Input: part model. Units: mm. Frame: model coordinates. A direction names the side the tool comes from. Coordinates: 2 decimals unless noted, no trailing zeros. Order: outer loops, then holes, each group sorted by start corner. A loop starts at its lowest first (then second) coordinate and runs counter-clockwise, first axis right, second up. Notation, with made-up numbers: M 19,-38 L 42,-38 A36 ccw 42,-2 Z; hole C -17.5,-22 d10. An arc over 180 degrees is marked long. One line per item, written item: value.
```python
from build123d import *

# Parameters (mm, degrees)
F0_W      = 55
F0_H      = 53.7
F0_R      = 2
F1_DEPTH  = 2
F2_DEPTH  = 4
F3_W      = 55
F3_H      = 27.5
F3_W_2    = 3.7
F3_H_2    = 2
F4_DEPTH  = 2
F5_START  = 1
F3_H_3    = 1.5
F5_DEPTH  = 1
F6_W      = 53.7
F6_H      = 27.5
F7_DEPTH  = 2
F8_START  = 1
F8_DEPTH  = 1
F10_DEPTH = 1.5
F11_W     = 55
F11_H     = 27.5
F11_W_2   = 3.7
F11_H_2   = 2
F12_DEPTH = 2
F13_START = 1
F13_DEPTH = 1
F15_DEPTH = 1.5
F16_W     = 1
F16_H     = 1.5
F16_W_2   = 53.7
F16_H_2   = 27.5
F17_DEPTH = 2
F18_START = 1
F18_DEPTH = 1
F20_DEPTH = 1.5
F21_W     = 1
F21_H     = 1
F22_DEPTH = 1.5
F23_R     = 0.3
F24_R     = 2
F25_R     = 0.5


with BuildPart() as f1:
    # F0 (on Top) → F1 (new body)
    with BuildSketch(Plane.XY):
        with Locations((27.5, 26.85)):
            Rectangle(F0_W, F0_H)
        with Locations((12, 11)):
            Circle(F0_R, mode=Mode.SUBTRACT)
        with Locations((43, 11)):
            Circle(F0_R, mode=Mode.SUBTRACT)
        with Locations((27.5, 46.7)):
            Circle(F0_R, mode=Mode.SUBTRACT)
    extrude(amount=F1_DEPTH)

    # F0 (on Top) → F2 (join)
    with BuildSketch(Plane.XY):
        with Locations((12, 11)):
            Circle(F0_R)
        with Locations((27.5, 46.7)):
            Circle(F0_R)
        with Locations((43, 11)):
            Circle(F0_R)
    extrude(amount=F2_DEPTH)

    # F3 (on face) → F4 (join)
    with BuildSketch(Plane.XZ):
        with Locations((27.5, 15.75)):
            Rectangle(F3_W, F3_H)
        with Locations((9.85, 26)):
            Rectangle(F3_W_2, F3_H_2, mode=Mode.SUBTRACT)
        with Locations((45.15, 26)):
            Rectangle(F3_W_2, F3_H_2, mode=Mode.SUBTRACT)
        with Locations((27.5, 1)):
            Rectangle(F3_W, F3_H_2)
    extrude(amount=F4_DEPTH)

    # F3 (on face) → F5 (join)
    with BuildSketch(Plane.XZ.offset(F5_START)):
        with Locations((27.5, 30.25)):
            Rectangle(F3_W, F3_H_3)
    extrude(amount=F5_DEPTH)

    # F6 (on face) → F7 (join)
    with BuildSketch(Plane.YZ.offset(55)):
        Polygon((-2, 29.5), (-2, 0), (53.7, 0), (53.7, 2), (0, 2), (0, 29.5), (-1, 29.5), align=None)
        with Locations((26.85, 15.75)):
            Rectangle(F6_W, F6_H)
        with BuildLine():
            ThreePointArc((23.7071067812, 9.7928932188), (22.2928932188, 9.7928932188), (22.2928932188, 11.2071067812))
            Line((22.2928932188, 11.2071067812), (32.2928932188, 21.2071067812))
            ThreePointArc((32.2928932188, 21.2071067812), (33.3826834324, 21.4238795325), (34, 20.5))
            ThreePointArc((34, 20.5), (33.9238795325, 20.1173165676), (33.7071067812, 19.7928932188))
            Line((33.7071067812, 19.7928932188), (23.7071067812, 9.7928932188))
        make_face(mode=Mode.SUBTRACT)
        with BuildLine():
            ThreePointArc((28.7071067812, 9.7928932188), (27.2928932188, 9.7928932188), (27.2928932188, 11.2071067812))
            Line((27.2928932188, 11.2071067812), (37.2928932188, 21.2071067812))
            ThreePointArc((37.2928932188, 21.2071067812), (38.3826834324, 21.4238795325), (39, 20.5))
            ThreePointArc((39, 20.5), (38.9238795325, 20.1173165676), (38.7071067812, 19.7928932188))
            Line((38.7071067812, 19.7928932188), (28.7071067812, 9.7928932188))
        make_face(mode=Mode.SUBTRACT)
        with BuildLine():
            ThreePointArc((33.7071067812, 9.7928932188), (32.2928932188, 9.7928932188), (32.2928932188, 11.2071067812))
            Line((32.2928932188, 11.2071067812), (42.2928932188, 21.2071067812))
            ThreePointArc((42.2928932188, 21.2071067812), (43.3826834324, 21.4238795325), (44, 20.5))
            ThreePointArc((44, 20.5), (43.9238795325, 20.1173165676), (43.7071067812, 19.7928932188))
            Line((43.7071067812, 19.7928932188), (33.7071067812, 9.7928932188))
        make_face(mode=Mode.SUBTRACT)
        with BuildLine():
            ThreePointArc((38.7071067812, 9.7928932188), (37.2928932188, 9.7928932188), (37.2928932188, 11.2071067812))
            Line((37.2928932188, 11.2071067812), (47.2928932188, 21.2071067812))
            ThreePointArc((47.2928932188, 21.2071067812), (48.3826834324, 21.4238795325), (49, 20.5))
            ThreePointArc((49, 20.5), (48.9238795325, 20.1173165676), (48.7071067812, 19.7928932188))
            Line((48.7071067812, 19.7928932188), (38.7071067812, 9.7928932188))
        make_face(mode=Mode.SUBTRACT)
    extrude(amount=F7_DEPTH)

    # F6 (on face) → F8 (join)
    with BuildSketch(Plane.YZ.offset(55).offset(F8_START)):
        Polygon((-1, 31), (-1, 29.5), (0, 29.5), (53.7, 29.5), (53.7, 31), align=None)
    extrude(amount=F8_DEPTH)

    # F9 (on face) → F10 (join)
    with BuildSketch(Plane.XY.offset(29.5)):
        Polygon((56, -1), (55, -1), (55, -2), (57, -2), (57, -1), align=None)
    extrude(amount=F10_DEPTH)

    # F11 (on face) → F12 (join)
    with BuildSketch(Plane(origin=(0, 53.7, 0), x_dir=(-1, 0, 0), z_dir=(0, 1, 0))):
        with Locations((-27.5, 15.75)):
            Rectangle(F11_W, F11_H)
        with Locations((-45.15, 26)):
            Rectangle(F11_W_2, F11_H_2, mode=Mode.SUBTRACT)
        with Locations((-9.85, 26)):
            Rectangle(F11_W_2, F11_H_2, mode=Mode.SUBTRACT)
        Polygon((-57, 29.5), (-57, 0), (0, 0), (0, 2), (-55, 2), (-55, 29.5), (-56, 29.5), align=None)
    extrude(amount=F12_DEPTH)

    # F11 (on face) → F13 (join)
    with BuildSketch(Plane(origin=(0, 53.7, 0), x_dir=(-1, 0, 0), z_dir=(0, 1, 0)).offset(F13_START)):
        Polygon((-56, 31), (-56, 29.5), (-55, 29.5), (0, 29.5), (0, 31), align=None)
    extrude(amount=F13_DEPTH)

    # F14 (on face) → F15 (join)
    with BuildSketch(Plane.XY.offset(29.5)):
        Polygon((56, 54.7), (56, 53.7), (57, 53.7), (57, 55.7), (56, 55.7), align=None)
    extrude(amount=F15_DEPTH)

    # F16 (on face) → F17 (join)
    with BuildSketch(Plane(origin=(0, 0, 0), x_dir=(0, -1, 0), z_dir=(-1, 0, 0))):
        Polygon((-55.7, 29.5), (-55.7, 0), (2, 0), (2, 29.5), (1, 29.5), (0, 29.5), (0, 2), (-53.7, 2), (-53.7, 29.5), (-54.7, 29.5), align=None)
        with Locations((1.5, 30.25)):
            Rectangle(F16_W, F16_H)
        with Locations((-26.85, 15.75)):
            Rectangle(F16_W_2, F16_H_2)
    extrude(amount=F17_DEPTH)

    # F16 (on face) → F18 (join)
    with BuildSketch(Plane(origin=(0, 0, 0), x_dir=(0, -1, 0), z_dir=(-1, 0, 0)).offset(F18_START)):
        Polygon((-54.7, 31), (-54.7, 29.5), (-53.7, 29.5), (0, 29.5), (1, 29.5), (1, 31), align=None)
    extrude(amount=F18_DEPTH)

    # F19 (on face) → F20 (join)
    with BuildSketch(Plane.XY.offset(29.5)):
        Polygon((0, 54.7), (0, 55.7), (-2, 55.7), (-2, 54.7), (-1, 54.7), align=None)
    extrude(amount=F20_DEPTH)

    # F21 (on face) → F22 (join)
    with BuildSketch(Plane.XY.offset(29.5)):
        with Locations((-0.5, -1.5)):
            Rectangle(F21_W, F21_H)
    extrude(amount=F22_DEPTH)

    # F23
    f23_edges = [f1.edges().sort_by_distance(p)[0] for p in [
        (8, -1, 27),
        (11.7, -1, 27),
        (8, -1, 25),
        (11.7, -1, 25),
        (43.3, -1, 25),
        (47, -1, 25),
        (43.3, -1, 27),
        (47, -1, 27),
        (47, 54.7, 27),
        (43.3, 54.7, 25),
        (43.3, 54.7, 27),
        (47, 54.7, 25),
        (11.7, 54.7, 25),
        (8, 54.7, 25),
        (11.7, 54.7, 27),
        (8, 54.7, 27),
    ]]
    fillet(f23_edges, radius=F23_R)

    # F24
    f24_edges = [f1.edges().sort_by_distance(p)[0] for p in [
        (57, 26.85, 0),
        (27.5, 55.7, 0),
        (27.5, -2, 0),
        (-2, 26.85, 0),
        (57, -2, 15.5),
        (57, 55.7, 15.5),
        (-2, 55.7, 15.5),
        (-2, -2, 15.5),
    ]]
    fillet(f24_edges, radius=F24_R)

    # F25
    f25_edges = [f1.edges().sort_by_distance(p)[0] for p in [
        (10, 11, 4),
        (25.5, 46.7, 4),
        (41, 11, 4),
    ]]
    fillet(f25_edges, radius=F25_R)


solid = f1.part
```
(1) Ray query, line 1 (Y direction, x = 47, z = 20.5); line 2 (X direction, y = 10.5, z = 8); line 3 (Z direction, x = 8.5, y = 18). Return the intervals inside material, ascending. Write a range as from..to.
Data:
line 1: y = -2..0, 53.7..55.7
line 2: x = -2..0, 55..57
line 3: z = 0..2
(2) Cut plane C-C on y = 35.5. Output: boundary loops of the cut face in (x, z), plus the area to 3 significant figures.
Data:
outline: M -2,2 A2 ccw 0,0 L 55,0 A2 ccw 57,2 L 57,11.59 L 55,11.59 L 55,2 L 0,2 L 0,29.5 L -1,29.5 L -1,31 L -2,31 Z; M 55,14.41 L 57,14.41 L 57,16.59 L 55,16.59 Z; M 55,19.41 L 57,19.41 L 57,31 L 56,31 L 56,29.5 L 55,29.5 Z
area: 218 mm2
(3) First-contact query: pin 1 (1.5 mm diameter, centred on y = 54.5, z = 26, fed in from +X); pin 2 (0.6 mm diameter, centred on x = 10, y = 54.5, fed in from -Z); pin 3 (1.5 mm diameter, centred on y = -1.5, z = 26, fed in from +X); pin 4 (1.5 mm diameter, centred on x = 12.5, y = 11.5, fed in from +Z). Flat tips, straight axial feed; report the tip coordinate or a pass-through.
Data:
pin 1: stops at x = 57
pin 2: stops at z = 0.06
pin 3: stops at x = 56.85
pin 4: stops at z = 4
(4) Cut plane B-B on x = 27.5. Output: boundary loops of the cut face in (y, z), plus the area to 3 significant figures.
Data:
outline: M -2,2 A2 ccw 0,0 L 53.7,0 A2 ccw 55.7,2 L 55.7,31 L 54.7,31 L 54.7,29.5 L 53.7,29.5 L 53.7,2 L 48.7,2 L 48.7,3.5 A0.5 ccw 48.2,4 L 45.2,4 A0.5 ccw 44.7,3.5 L 44.7,2 L 0,2 L 0,29.5 L -1,29.5 L -1,31 L -2,31 Z
area: 235 mm2
(5) Draft query along X for faces 1 (the flat face through (45, -1, 27)), 2 (the cylindrical face through (56.4, -1.43, 16.7)), 3 (the flat face through (28, 27, 0)). Return one class per face: released by +X, released by -X, zero draft, split by the parting line, or undercut.
Data:
face 1: undercut
face 2: released by +X
face 3: zero draft
(6) Cut plane D-D on z = 17. Output: boundary loops of the cut face in (x, y), plus the area to 3 significant figures.
Data:
outline: M -2,0 A2 ccw 0,-2 L 55,-2 A2 ccw 57,0 L 57,28.09 L 55,28.09 L 55,0 L 0,0 L 0,53.7 L 55,53.7 L 55,45.91 L 57,45.91 L 57,53.7 A2 ccw 55,55.7 L 0,55.7 A2 ccw -2,53.7 Z; M 55,30.91 L 57,30.91 L 57,33.09 L 55,33.09 Z; M 55,35.91 L 57,35.91 L 57,38.09 L 55,38.09 Z; M 55,40.91 L 57,40.91 L 57,43.09 L 55,43.09 Z
area: 425 mm2
(7) Access query for faces 4 (the cylindrical face through (55.986, 27.309, 9.778)), 5 (the flat face through (0, 27, 16)), 6 (the flat face through (43.3, 55, 26)). Directions: +Z, -Z, +X, -X, +Y, -Y. A direction counts if a zero-diameter tool reaches every point of the face in a straight line with its end or side. Return the directions, or none.
Data:
face 4: +X
face 5: +Z
face 6: +Y, -Y
(8) Cut plane A-A on y = 23. Output: boundary loops of the cut face in (x, z), plus the area to 3 significant figures.
Data:
outline: M -2,2 A2 ccw 0,0 L 55,0 A2 ccw 57,2 L 57,9.5 L 55,9.5 L 55,2 L 0,2 L 0,29.5 L -1,29.5 L -1,31 L -2,31 Z; M 55,11.91 L 57,11.91 L 57,31 L 56,31 L 56,29.5 L 55,29.5 Z
area: 224 mm2
